Design review of the part built by this model. Coordinates are the model's own, in mm. Give positions to 0.01 mm unless a question says otherwise; leave off trailing zeros. Order: outer loops, then holes, each group sorted by start corner. A loop starts at its lowest first (then second) coordinate and runs counter-clockwise, first axis right, second up. Notation, with made-up numbers: (56, -2.75) -> (111, -2.75) arc R20 cw to (111, 8.25) -> close; hole circle Ø8 at (57.5, -11). An arc over 180 degrees is marked (long way). One line per item, written item: value.
Autodesk Inventor part; units mm, degrees
ref_plane "YZ Plane" through (0, 0, 0) normal (1, 0, 0) x (0, 1, 0)
ref_plane "XZ Plane" through (0, 0, 0) normal (0, 1, 0) x (-1, 0, 0)
ref_plane "XY Plane" through (0, 0, 0) normal (0, 0, 1) x (1, 0, 0)
sketch "スケッチ1" plane through (0, 0, 0) normal (0, 0, 1) x (1, 0, 0)
  circle A0 centre (0, 0) radius 47.6
  circle A1 centre (0, 0) radius 67.5
  dimension "d0" = 95.2
  dimension "d1" = 135
extrude "押し出し1" add sketch "スケッチ1" along normal blind 10
sketch "スケッチ2" plane through (0, 0, 10) normal (0, 0, 1) x (1, 0, 0)
  circle A0 centre (0, 0) radius 62.5
  point P0 (16.1762, 60.3704)
  point P1 (-16.1762, 60.3704)
  point P2 (-44.1942, 44.1942)
  point P3 (-60.3704, 16.1762)
  point P4 (-60.3704, -16.1762)
  point P5 (-44.1942, -44.1942)
  point P6 (-16.1762, -60.3704)
  point P7 (16.1762, -60.3704)
  point P8 (44.1942, -44.1942)
  point P9 (60.3704, -16.1762)
  point P10 (60.3704, 16.1762)
  point P11 (44.1942, 44.1942)
  dimension "d4" = 125
  dimension "d7" = 360
  dimension "d25" = 0
hole "穴1" at (16.1762, 60.3704, 10) at (-16.1762, 60.3704, 10) at (-44.1942, 44.1942, 10) at (-60.3704, 16.1762, 10) at (-60.3704, -16.1762, 10) at (-44.1942, -44.1942, 10) at (-16.1762, -60.3704, 10) at (16.1762, -60.3704, 10) at (44.1942, -44.1942, 10) at (60.3704, -16.1762, 10) at (60.3704, 16.1762, 10) at (44.1942, 44.1942, 10) direction (0, 0, -1) diameter 4.3 end through all
chamfer "面取り1" distance 1 angle 45 2 edges at (-47.6, 0, 10) (-47.6, 0, 0)
sketch "スケッチ3" plane through (0, 0, 10) normal (0, 0, 1) x (1, 0, 0)
  circle A0 centre (16.1762, 60.3704) radius 2.15
  circle A1 centre (-16.1762, 60.3704) radius 2.15
  circle A2 centre (0, 0) radius 67.5
  circle A3 centre (0, 0) radius 62.5
  circle A4 centre (-16.1762, 60.3704) radius 5
  circle A5 centre (16.1762, 60.3704) radius 5
  point P0 (11.2987, 61.4702)
  point P1 (17.4703, 65.2)
  point P2 (-17.4703, 65.2)
  point P3 (-20.9502, 58.8841)
properties part number "unit-j2-base2" material "ABS プラスチック"
Item 1: Clearance check with flat-ended pins moving along their axes: P1, Ø3, axis at x = -8, z = 7.5, coming from the +Y side; P2, Ø5, axis at y = -5, z = 6.5, coming from the -X side; P3, Ø3, axis at y = -42, z = 6, coming from the +X side. State where each tip first meets the part, or that it passes through.
Returned:
P1: y = 67.19
P2: x = -67.45
P3: x = 54
Item 2: Add section D-D on y = -54. Give the boundary of the cut face in (x, z).
Returned:
outline: (-40.5, 0) -> (40.5, 0) -> (40.5, 10) -> (-40.5, 10) -> close
Item 3: Add section C-C on z = 6.25. Count the separate pieces of the cut face and the enclosed holes in it, plus the area to 3 significant figures.
Returned:
separate pieces: 1
enclosed holes: 13
area: 7,020 mm²
Item 4: Add section A-A on y = 0. Give the boundary of the cut face in (x, z).
Returned:
outline: (-67.5, 0) -> (-48.6, 0) -> (-47.6, 1) -> (-47.6, 9) -> (-48.6, 10) -> (-67.5, 10) -> close; (47.6, 1) -> (48.6, 0) -> (67.5, 0) -> (67.5, 10) -> (48.6, 10) -> (47.6, 9) -> close
Item 5: To check wall thickness, follow line 1 along Y through (x, z) = (58.5, 4.25); line 2 along Y through (x, z) = (62, 6); line 3 along Y through (x, z) = (0, 5.75). State the ranges of each line that lie inside material, in increasing order. Write a range as from..to.
Returned:
line 1: -33.67..-17.24, -15.12..15.12, 17.24..33.67
line 2: -26.69..-17.58, -14.77..14.77, 17.58..26.69
line 3: -67.5..-47.6, 47.6..67.5
Item 6: Draft analysis for pull direction X (two halves, no side actions). For faces 1 (the cylindrical face through (-53.57, 41.07, 4.93)), 2 (the flat face through (45, 20, 0)), 3 (the cylindrical face through (-45.65, -42.61, 4.93)), state which applies: pulls with the +X half, pulls with the -X half, needs draft (parallel to the pull), parting line crosses it, or undercut.
Returned:
face 1: parting line crosses it
face 2: needs draft
face 3: undercut
